from build123d import *

# Parameters (mm, degrees)
SKETCH1_W           = 150
SKETCH1_H           = 60
BOSS_EXTRUDE1_DEPTH = 3
FILLET1_R           = 30
SKETCH2_W           = 89.6
SKETCH2_H           = 20
BOSS_EXTRUDE2_DEPTH = 3
FILLET2_R           = 30
SKETCH3_R           = 0.8
SKETCH3_R_2         = 0.899402105
CUT_EXTRUDE1_DEPTH  = 154.407952858
FILLET3_R           = 5
SKETCH4_W           = 20
SKETCH4_H           = 100
BOSS_EXTRUDE3_DEPTH = 3
BOSS_EXTRUDE4_DEPTH = 3


with BuildPart() as part:
    # Sketch1 → Boss-Extrude1 (new body)
    with BuildSketch(Plane(origin=(0, 0, 0), x_dir=(1, 0, 0), z_dir=(0, 1, 0))):
        Rectangle(SKETCH1_W, SKETCH1_H)
    extrude(amount=BOSS_EXTRUDE1_DEPTH)

    # Fillet1
    fillet1_edges = [part.edges().sort_by_distance(p)[0] for p in [
        (75, 1.5, 30),
    ]]
    fillet(fillet1_edges, radius=FILLET1_R)

    # Sketch2 → Boss-Extrude2 (add)
    with BuildSketch(Plane(origin=(0, 3, 0), x_dir=(1, 0, 0), z_dir=(0, 1, 0))):
        Polygon((-75, 30), (-55, 30), (-55, 50), (-145, 50), (-145, 30), align=None)
        Polygon((-75, -30), (-75, 30), (-145, 30), align=None)
        with Locations((10, 40)):
            Rectangle(SKETCH2_W, SKETCH2_H)
    extrude(amount=-BOSS_EXTRUDE2_DEPTH)

    # Fillet2
    fillet2_edges = [part.edges().sort_by_distance(p)[0] for p in [
        (-145, 1.5, -30),
        (-75, 1.5, 30),
    ]]
    fillet(fillet2_edges, radius=FILLET2_R)

    # Sketch3 → Cut-Extrude1 (cut, through all)
    with BuildSketch(Plane(origin=(0, 3, 0), x_dir=(1, 0, 0), z_dir=(0, 1, 0))):
        with Locations((-55, 30)):
            Circle(SKETCH3_R)
        with Locations((-34.8, 30)):
            Circle(SKETCH3_R)
        with Locations((54.8, 30)):
            Circle(SKETCH3_R_2)
    extrude(amount=-CUT_EXTRUDE1_DEPTH, mode=Mode.SUBTRACT)

    # Fillet3
    fillet3_edges = [part.edges().sort_by_distance(p)[0] for p in [
        (-34.8, 1.5, -50),
        (54.8, 1.5, -50),
        (75, 1.5, -30),
    ]]
    fillet(fillet3_edges, radius=FILLET3_R)

    # Sketch4 → Boss-Extrude3 (add)
    with BuildSketch(Plane(origin=(0, 0, 0), x_dir=(-1, 0, 0), z_dir=(0, -1, 0))):
        with Locations((135, 100)):
            Rectangle(SKETCH4_W, SKETCH4_H)
    extrude(amount=-BOSS_EXTRUDE3_DEPTH)

    # Sketch5 → Boss-Extrude4 (add)
    with BuildSketch(Plane(origin=(0, 3, 0), x_dir=(1, 0, 0), z_dir=(0, 1, 0))):
        Polygon((-55, 50), (-125, 50), (-125, 150), (-95, 150), (-55, 126.905989232), align=None)
    extrude(amount=-BOSS_EXTRUDE4_DEPTH)


solid = part.part
Work out the finished part from the listing and answer in its coordinate system (mm). Round coordinates to 2 decimals unless told otherwise and drop trailing zeros. Order: outer loops, then holes, each group sorted by start corner. A loop starts at its lowest first (then second) coordinate and runs counter-clockwise, first axis right, second up. Notation, with made-up numbers: M -4.75,78.25 L 35.25,78.25 A17 ccw 35.25,94.25 Z; hole C -6,-24 d9. An arc over 180 degrees is marked long. Put each result on its own line as item: value. Start each with the question number.
Q1. Section C-C, the plane x = -50.5 is taken. Write down the section's boundary in (y, z), and give its area (3 significant figures).
Q2. For a pull along X with two mould halves and no side action, classify faces 1 (the flat face through (-109.3, 1.5, 0.6)), 2 (the cylindrical face through (-33.37, 1.48, -48.5)), 3 (the cylindrical face through (65.979, 1.521, 21.445)), 4 (the flat face through (-58, 0, -41)) as pulls with the +X half, pulls with the -X half, needs draft (parallel to the pull), parting line crosses it, or undercut.
Q3. Straight lines are drawn through the part: L1, parallel to X at y = 2.3, z = -60; L2, parallel to X at y = 1.2, z = -46; L3, parallel to Z at x = 15, y = 2.95. For each, find the intervals that lie inside material, in ascending order. Write a range as [from, to].
Q4. Section B-B, the plane y = 1.55 is taken. Write down the section's boundary in (x, z).
Q5. Flat-ended cylindrical pins translate along their axes: pin 1 (1.5 mm diameter, centred on y = 2, z = -38.5, fed in from -X); pin 2 (1.5 mm diameter, centred on x = -48.5, y = 1.5, fed in from -Z); pin 3 (0.9 mm diameter, centred on x = 5.5, y = 1.5, fed in from -Z). Find the tip coordinate at first contact, or state that the pin passes through.
Q6. Section A-A, the plane z = -35 is taken. Write down the section's boundary in (x, y).
Q7. Section D-D, the plane z = -112.5 is taken. Write down the section's boundary in (x, y), and give its area (3 significant figures).
Findings below:
1. outline: M 0,-30 L 3,-30 L 3,30 L 0,30 Z
1. area: 180 mm^2
2. face 1: pulls with the -X half
2. face 2: undercut
2. face 3: pulls with the +X half
2. face 4: needs draft
3. L1: x = [-145, -55]
3. L2: x = [-145, -55], [-34.7, 54.7]
3. L3: z = [-50, 30]
4. outline: M -145,-150 L -95,-150 L -55,-126.91 L -55,-30.8 A0.8 cw long -54.2,-30 L -35.6,-30 A0.8 cw long -34.8,-30.8 L -34.8,-45 A5 ccw -29.8,-50 L 49.8,-50 A5 ccw 54.8,-45 L 54.8,-30.9 A0.9 cw long 55.7,-30 L 70,-30 A5 ccw 75,-25 L 75,0 A30 ccw 45,30 L -63.9,30 A30 ccw -83.43,22.78 L -134.52,-21.02 A30 ccw -145,-43.8 Z
5. pin 1: stops at x = -144.65
5. pin 2: stops at z = -30
5. pin 3: stops at z = -50
6. outline: M -143.68,0 L -55,0 L -55,3 L -143.68,3 Z; M -34.8,0 L 54.8,0 L 54.8,3 L -34.8,3 Z
7. outline: M -145,0 L -55,0 L -55,3 L -145,3 Z
7. area: 270 mm^2
